```python
from build123d import *

# Parameters (mm, degrees)
F5_DEPTH       = 40
F1_D           = 3.5
F7_D           = 23
F2_D           = 5.5
F2_CBORE_D     = 10
F2_CBORE_DEPTH = 2
F3_R           = 5
F4_R           = 1


with BuildPart() as f5:
    # F0 (on Top) → F5 (new body)
    with BuildSketch(Plane.XY):
        Polygon((0, 23.38951), (0, -29.61049), (4, -29.61049), (4, 17.38951), (24, 17.38951), (24, 23.38951), align=None)
    extrude(amount=F5_DEPTH)

    # F1 (through all)
    with Locations(Plane.YZ.offset(4)):
        with Locations((-21.61049, 35.5), (9.38951, 35.5), (-21.61049, 4.5), (9.38951, 4.5)):
            Hole(F1_D / 2)

    # F7 (through all)
    with Locations(Plane.YZ.offset(4)):
        with Locations((-6.11049, 20)):
            Hole(F7_D / 2)

    # F2 (through all)
    with Locations(Plane.XZ.offset(-17.38951)):
        with Locations((14, 30), (14, 10)):
            CounterBoreHole(F2_D / 2, F2_CBORE_D / 2, F2_CBORE_DEPTH)

    # F3
    f3_edges = [f5.edges().sort_by_distance(p)[0] for p in [
        (2, -29.61049, 40),
        (2, -29.61049, 0),
        (24, 20.38951, 40),
        (24, 20.38951, 0),
    ]]
    fillet(f3_edges, radius=F3_R)

    # F4
    f4_edges = [f5.edges().sort_by_distance(p)[0] for p in [
        (0, 23.38951, 20),
    ]]
    fillet(f4_edges, radius=F4_R)


solid = f5.part
```
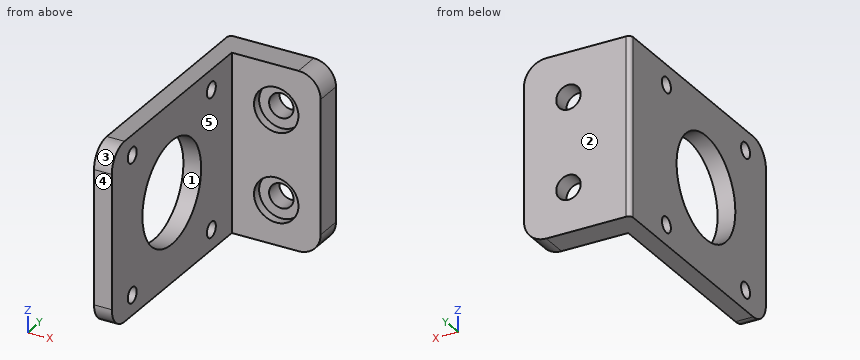
For this review, take the finished solid that the model builds, in its own axes (mm). Face numbers are marked on the shaded views. A direction names the side the tool comes from. Coordinates: 2 decimals unless noted, no trailing zeros. Write each loop counter-clockwise with the first axis right and the second up, starting at its lowest first coordinate (ties: lowest second). Pieces come first, ordered by that corner, then holes. Notation, with made-up numbers: (19.25, 66) - (26.25, 66) arc R27 ccw to (26.25, 85) - close; hole circle Ø9 at (10.25, 63.25). An arc over 180 degrees is marked (long way). Answer in a Markdown table with one row per item. Add a question column.
Q1. For probe 1 along Z at (x, y) = (14, 18.9); probe 2 along Y at (x, z) = (9.5, 34.5); probe 3 along X at (y, z) = (0, 30.5), list the stretches that pass through material, from the lowest coordinate up.
Q2. We need section C-C, the plane y = -4. State the section outline as (x, z) points.
Q3. We need section A-A, the plane x = 14. State the section outline as (y, z) points.
Q4. Draft analysis for pull direction Z (two halves, no side actions). For the marked faces 1, 2 and 3, state which applies: +Z half, -Z half, draft (parallel to the pull), parting line (faces both ways), or undercut.
Q5. For P1, Ø10, axis at x = 16, z = 25.5, coming from the -Y side; P2, Ø10, axis at y = 8, z = 33.5, coming from the -X side; P3, Ø3, axis at x = 14.5, z = 11.5, coming from the -Y side, all flat-tipped, find the tip position at first contact; note any pin that passes through.
Q6. We need section D-D, the plane z = 10. State the section outline as (x, y) points, and give its area (3 significant figures).
Q7. We need section B-B, the plane z = 20. State the section outline as (x, y) points.
Q8. Tool access review of the marked faces 4 and 5: name each direction out of +Z, -Z, +X, -X, +Y, -Y from which nothing blocks a thin tool from reaching the whole face with its end or side.
Answer list:
| question | item | result |
|---|---|---|
| 1 | probe 1 | z = 0 to 5, 15 to 25, 35 to 40 |
| 1 | probe 2 | y = 17.39 to 23.39 |
| 1 | probe 3 | x = 0 to 4 |
| 2 | outline | (0, 0) - (4, 0) - (4, 8.7) - (0, 8.7) - close; (0, 31.3) - (4, 31.3) - (4, 40) - (0, 40) - close |
| 3 | outline | (17.39, 0) - (23.39, 0) - (23.39, 7.25) - (19.39, 7.25) - (19.39, 5) - (17.39, 5) - close; (17.39, 15) - (19.39, 15) - (19.39, 12.75) - (23.39, 12.75) - (23.39, 27.25) - (19.39, 27.25) - (19.39, 25) - (17.39, 25) - close; (17.39, 35) - (19.39, 35) - (19.39, 32.75) - (23.39, 32.75) - (23.39, 40) - (17.39, 40) - close |
| 4 | face 1 | undercut |
| 4 | face 2 | draft |
| 4 | face 3 | +Z half |
| 5 | P1 | stops at y = 17.39 |
| 5 | P2 | stops at x = 0 |
| 5 | P3 | stops at y = 19.39 |
| 6 | outline | (0, -29.61) - (4, -29.61) - (4, -11.79) - (0, -11.79) - close; (0, -0.43) - (4, -0.43) - (4, 17.39) - (9, 17.39) - (9, 19.39) - (11.25, 19.39) - (11.25, 23.39) - (1, 23.39) arc R1 ccw to (0, 22.39) - close; (16.75, 19.39) - (19, 19.39) - (19, 17.39) - (24, 17.39) - (24, 23.39) - (16.75, 23.39) - close |
| 6 | area | 244 mm2 |
| 7 | outline | (0, -29.61) - (4, -29.61) - (4, -17.61) - (0, -17.61) - close; (0, 5.39) - (4, 5.39) - (4, 17.39) - (24, 17.39) - (24, 23.39) - (1, 23.39) arc R1 ccw to (0, 22.39) - close |
| 8 | face 4 | +Z, -Z, +X, -X, -Y |
| 8 | face 5 | +Z, -Z, +X, -Y |
